Here's the drawing with two shaded views (mm, measured from the low corner). I have some questions. A direction names the side the tool comes from. Coordinates: 2 decimals unless noted, no trailing zeros. Write each loop counter-clockwise with the first axis right and the second up, starting at its lowest first coordinate (ties: lowest second). Pieces come first, ordered by that corner, then holes.
Item 1: I want a section at B-B on x = 38. Please give me the cut outline in (y, z), then the cut area to 3 significant figures.
Item 2: Which directions (+Z, -Z, +X, -X, +Y, -Y) give clear straight access to the entire face, cutting with the end or side of a thin tool? Please do the marked faces 1, 2, 3, 4 and 5.
Item 3: For P1, Ø0.5, axis at y = 4, z = 2.5, coming from the +X side; P2, Ø3, axis at y = 3, z = 11, coming from the -X side; P3, Ø3, axis at x = 4, y = 4, coming from the +Z side; P4, Ø1.8, axis at x = 29.45, z = 9, coming from the +Y side, each with a flat end and sliding along its axis, tell me the tip position at first contact or that it passes through.
Item 4: I want a section at A-A on y = 5.6. Please give me the cut outline in (x, z).
Item 5: Thinking about a two-plate mould opening in Z: for the marked faces 6, 7, 8 and 9, which applies, +Z half, -Z half, draft (parallel to the pull), parting line (faces both ways), or undercut?
Item 6: I want a section at C-C on z = 9.5. Please give me the cut outline in (x, y), then the cut area to 3 significant figures.
Item 7: I want a section at D-D on y = 2.2. Please give me the cut outline in (x, z), then the cut area to 3 significant figures.
Item 8: If I drill on probe 1 along X at (y, z) = (1.4, 9); probe 2 along X at (y, z) = (4.7, 9); probe 3 along Y at (x, z) = (3, 3.6), over which ranges is the centre line in solid material (lowest first)?
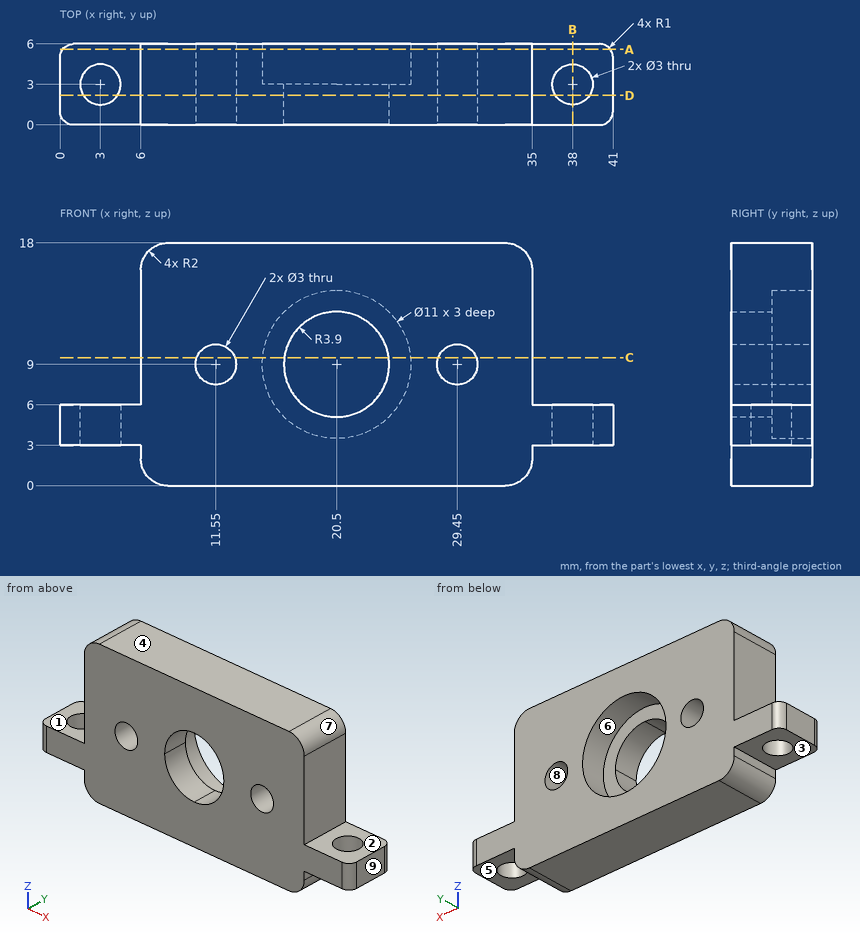
Response values:
1. outline: (0, 3) - (1.5, 3) - (1.5, 6) - (0, 6) - close; (4.5, 3) - (6, 3) - (6, 6) - (4.5, 6) - close
1. area: 9.00 mm2
2. face 1: +Z, -X, +Y, -Y
2. face 2: +Z, +X, +Y, -Y
2. face 3: -Z, -X, +Y, -Y
2. face 4: +Z, +X, -X, +Y, -Y
2. face 5: -Z, +X, +Y, -Y
3. P1: stops at x = 35
3. P2: stops at x = 6
3. P3: stops at z = 6
3. P4: passes through
4. outline: (0.2, 3) - (6, 3) - (6, 2) arc R2 ccw to (8, 0) - (33, 0) arc R2 ccw to (35, 2) - (35, 3) - (40.8, 3) - (40.8, 6) - (35, 6) - (35, 16) arc R2 ccw to (33, 18) - (8, 18) arc R2 ccw to (6, 16) - (6, 6) - (0.2, 6) - close; hole circle Ø3 at (11.55, 9); hole circle Ø11 at (20.5, 9); hole circle Ø3 at (29.45, 9)
5. face 6: undercut
5. face 7: +Z half
5. face 8: undercut
5. face 9: draft
6. outline: (6, 0) - (10.14, 0) - (10.14, 6) - (6, 6) - close; (12.96, 0) - (16.63, 0) - (16.63, 3) - (15.02, 3) - (15.02, 6) - (12.96, 6) - close; (24.37, 0) - (28.04, 0) - (28.04, 6) - (25.98, 6) - (25.98, 3) - (24.37, 3) - close; (30.86, 0) - (35, 0) - (35, 6) - (30.86, 6) - close
6. area: 84.0 mm2
7. outline: (0, 3) - (1.73, 3) - (1.73, 6) - (0, 6) - close; (4.27, 3) - (6, 3) - (6, 2) arc R2 ccw to (8, 0) - (33, 0) arc R2 ccw to (35, 2) - (35, 3) - (36.73, 3) - (36.73, 6) - (35, 6) - (35, 16) arc R2 ccw to (33, 18) - (8, 18) arc R2 ccw to (6, 16) - (6, 6) - (4.27, 6) - close; (39.27, 3) - (41, 3) - (41, 6) - (39.27, 6) - close; hole circle Ø3 at (11.55, 9); hole circle Ø7.8 at (20.5, 9); hole circle Ø3 at (29.45, 9)
7. area: 477 mm2
8. probe 1: x = 6 to 10.05, 13.05 to 16.6, 24.4 to 27.95, 30.95 to 35
8. probe 2: x = 6 to 10.05, 13.05 to 15, 26 to 27.95, 30.95 to 35
8. probe 3: y = 0 to 1.5, 4.5 to 6
